For this review, take the finished solid that the model builds, in its own axes (mm). A direction names the side the tool comes from. Coordinates: 2 decimals unless noted, no trailing zeros. Loops run counter-clockwise (first coordinate to the right, second up) from the corner with the lowest first, then second, coordinate; pieces in that order, holes last. Notation, with made-up numbers: M 69.5,19.25 L 73.5,19.25 A22 cw 73.5,38.25 Z; hole C 87.25,-1 d5. An arc over 180 degrees is marked long. Write each question's results on one line, items separated by ' | '. Start each with the question number.
```python
from build123d import *

# Parameters (mm, degrees)
F1_DEPTH = 50
F2_DEPTH = 50
F3_DEPTH = 50


with BuildPart() as f1:
    # F0 (on Top) → F1 (new body)
    with BuildSketch(Plane.XY):
        Polygon((-38, -32.4384031666), (0, -32.4384031666), (38, -32.4384031666), (36, 0), (0, 0), (-36, 0), align=None)
    extrude(amount=F1_DEPTH)

    # F2 (add): a face of the model
    f2_faces = [f1.faces().sort_by_distance(p)[0] for p in [
        (0, 0, 25),
    ]]
    extrude(f2_faces, amount=F2_DEPTH)

    # F3 (add): a face of the model
    f3_faces = [f1.faces().sort_by_distance(p)[0] for p in [
        (0, -32.4384031666, 25),
    ]]
    extrude(f3_faces, amount=F3_DEPTH)


solid = f1.part
```
Q1. Take a section at C-C, the plane y = -9.5. Give the boundary of the cut face in (x, z).
Q2. To check wall thickness, follow line 1 along X through (y, z) = (43, 37); line 2 along X through (y, z) = (-7.5, 28). State the ranges of each line that lie inside material, in increasing order.
Q3. Take a section at A-A, the plane z = 19. Give the boundary of the cut face in (x, y), then the cut area to 3 significant figures.
Q4. Take a section at B-B, the plane y = 4.5. Give the boundary of the cut face in (x, z), then the cut area to 3 significant figures.
Q5. For faces 1 (the face through (-36, 25, 25)), 2 (the face through (-38, -57, 25)), 3 (the face through (36, 25, 25)), list the 3-axis set-ups (+Z, -Z, +X, -X, +Y, -Y) from which the entire face can be reached by the end or side of a thin tool; tool diameter is ignored.
Q6. Insertion check: P1, Ø25, axis at y = 29.5, z = 24.5, coming from the +X side; P2, Ø12, axis at y = 25, z = 10.5, coming from the -X side; P3, Ø12, axis at y = -21.5, z = 11.5, coming from the +X side. Each pin has a flat end and moves straight along its axis. Give the tip position at first contact, or say it passes through.
Results:
1) outline: M -36.59,0 L 36.59,0 L 36.59,50 L -36.59,50 Z
2) line 1: -36 to 36 | line 2: -36.46 to 36.46
3) outline: M -38,-82.44 L 38,-82.44 L 38,-32.44 L 36,0 L 36,50 L -36,50 L -36,0 L -38,-32.44 Z | area: 9,800 mm^2
4) outline: M -36,0 L 36,0 L 36,50 L -36,50 Z | area: 3,600 mm^2
5) face 1: +Z, -Z, -X, +Y | face 2: +Z, -Z, -X, +Y, -Y | face 3: +Z, -Z, +X, +Y
6) P1: x = 36 | P2: x = -36 | P3: x = 37.7
